```python
from build123d import *

# Parameters (mm, degrees)
BOSS_EXTRUDE1_DEPTH      = 15
BOSS_EXTRUDE1_DEPTH_BACK = 22.5
SKETCH2_W                = 240
SKETCH2_H                = 40
CUT_EXTRUDE1_REACH       = 130.477
SKETCH3_W                = 16
SKETCH3_H                = 2.2
SKETCH3_H_2              = 2.5
SKETCH5_W                = 240
SKETCH5_H                = 40
CUT_EXTRUDE2_DEPTH       = 8
SKETCH6_W                = 20
SKETCH6_H                = 30
BOSS_EXTRUDE2_DEPTH      = 75
CUT_EXTRUDE3_REACH       = 161.707
SKETCH8_W                = 10
SKETCH8_H                = 4.8
SKETCH8_H_2              = 4.5
SKETCH9_R                = 2.1
CUT_EXTRUDE4_DEPTH       = 4.4
SKETCH11_R               = 1.55
CUT_EXTRUDE5_DEPTH       = 11
SKETCH10_R               = 1.55
CUT_EXTRUDE6_DEPTH       = 11
SKETCH12_R               = 2.1
CUT_EXTRUDE7_DEPTH       = 4.4
SKETCH13_R               = 1.65
CUT_EXTRUDE8_DEPTH       = 11
SKETCH14_W               = 18
SKETCH14_H               = 12
CUT_EXTRUDE9_DEPTH       = 29.5
SKETCH15_W               = 10
SKETCH15_H               = 14
CUT_EXTRUDE10_DEPTH      = 20
BOSS_EXTRUDE3_DEPTH      = 10
BOSS_EXTRUDE3_DEPTH_BACK = 50
CUT_EXTRUDE11_REACH      = 163.927
SKETCH18_W               = 89.999903017
SKETCH18_H               = 5
SKETCH18_W_2             = 6.000219265
SKETCH18_W_3             = 65.999877718
SKETCH20_W               = 11
SKETCH20_H               = 12
CUT_EXTRUDE12_DEPTH      = 7
SKETCH21_W               = 8
SKETCH21_H               = 0.5
CUT_EXTRUDE13_DEPTH      = 2
SKETCH22_W               = 8
SKETCH22_H               = 1
CUT_EXTRUDE14_DEPTH      = 2
CUT_EXTRUDE15_REACH      = 163.927
SKETCH23_W               = 11
SKETCH23_H               = 8


with BuildPart() as part:
    # Sketch2 → Boss-Extrude1 (new, two sides: drawn at the far end of the back side and taken through both)
    with BuildSketch(Plane(origin=(0, 0, 0), x_dir=(1, 0, 0), z_dir=(0, 1, 0)).offset(-BOSS_EXTRUDE1_DEPTH_BACK)):
        Rectangle(SKETCH2_W, SKETCH2_H)
    extrude(amount=BOSS_EXTRUDE1_DEPTH + BOSS_EXTRUDE1_DEPTH_BACK)

    # Sketch3 → Cut-Extrude1 (cut, up to next)
    with BuildSketch(Plane.XY.offset(20), mode=Mode.PRIVATE) as cut_extrude1_sk1:
        with Locations((-107, 1.1)):
            Rectangle(SKETCH3_W, SKETCH3_H)
    cut_extrude1_tool1 = extrude(cut_extrude1_sk1.sketch, amount=-CUT_EXTRUDE1_REACH, mode=Mode.PRIVATE) & part.part
    # Sketch3 → Cut-Extrude1 (cut, up to next)
    with BuildSketch(Plane.XY.offset(20), mode=Mode.PRIVATE) as cut_extrude1_sk2:
        with Locations((8.999903017, 1.25)):
            Rectangle(SKETCH3_W, SKETCH3_H_2)
    cut_extrude1_tool2 = extrude(cut_extrude1_sk2.sketch, amount=-CUT_EXTRUDE1_REACH, mode=Mode.PRIVATE) & part.part
    # Sketch3 → Cut-Extrude1 (cut, up to next)
    with BuildSketch(Plane.XY.offset(20), mode=Mode.PRIVATE) as cut_extrude1_sk3:
        with Locations((100.999780735, 1.1)):
            Rectangle(SKETCH3_W, SKETCH3_H)
    cut_extrude1_tool3 = extrude(cut_extrude1_sk3.sketch, amount=-CUT_EXTRUDE1_REACH, mode=Mode.PRIVATE) & part.part
    add(cut_extrude1_tool1.solids().sort_by_distance((-107, 1.1, 20))[0], mode=Mode.SUBTRACT)
    add(cut_extrude1_tool2.solids().sort_by_distance((8.999903, 1.25, 20))[0], mode=Mode.SUBTRACT)
    add(cut_extrude1_tool3.solids().sort_by_distance((100.999781, 1.1, 20))[0], mode=Mode.SUBTRACT)

    # Sketch5 → Cut-Extrude2 (cut)
    with BuildSketch(Plane(origin=(0, 15, 0), x_dir=(1, 0, 0), z_dir=(0, 1, 0))):
        Rectangle(SKETCH5_W, SKETCH5_H)
    extrude(amount=-CUT_EXTRUDE2_DEPTH, mode=Mode.SUBTRACT)

    # Sketch6 → Boss-Extrude2 (add)
    with BuildSketch(Plane.XZ.offset(22.5)):
        with Locations((-70, 0)):
            Rectangle(SKETCH6_W, SKETCH6_H)
    extrude(amount=BOSS_EXTRUDE2_DEPTH)

    # Sketch8 → Cut-Extrude3 (cut, up to next)
    with BuildSketch(Plane.XY.offset(20), mode=Mode.PRIVATE) as cut_extrude3_sk1:
        with Locations((-107, 4.6)):
            Rectangle(SKETCH8_W, SKETCH8_H)
    cut_extrude3_tool1 = extrude(cut_extrude3_sk1.sketch, amount=-CUT_EXTRUDE3_REACH, mode=Mode.PRIVATE) & part.part
    # Sketch8 → Cut-Extrude3 (cut, up to next)
    with BuildSketch(Plane.XY.offset(20), mode=Mode.PRIVATE) as cut_extrude3_sk2:
        with Locations((8.999903017, 4.75)):
            Rectangle(SKETCH8_W, SKETCH8_H_2)
    cut_extrude3_tool2 = extrude(cut_extrude3_sk2.sketch, amount=-CUT_EXTRUDE3_REACH, mode=Mode.PRIVATE) & part.part
    # Sketch8 → Cut-Extrude3 (cut, up to next)
    with BuildSketch(Plane.XY.offset(20), mode=Mode.PRIVATE) as cut_extrude3_sk3:
        with Locations((100.999780735, 4.6)):
            Rectangle(SKETCH8_W, SKETCH8_H)
    cut_extrude3_tool3 = extrude(cut_extrude3_sk3.sketch, amount=-CUT_EXTRUDE3_REACH, mode=Mode.PRIVATE) & part.part
    add(cut_extrude3_tool1.solids().sort_by_distance((-107, 4.6, 20))[0], mode=Mode.SUBTRACT)
    add(cut_extrude3_tool2.solids().sort_by_distance((8.999903, 4.75, 20))[0], mode=Mode.SUBTRACT)
    add(cut_extrude3_tool3.solids().sort_by_distance((100.999781, 4.6, 20))[0], mode=Mode.SUBTRACT)

    # Sketch9 → Cut-Extrude4 (cut)
    with BuildSketch(Plane(origin=(0, 0, 0), x_dir=(1, 0, 0), z_dir=(0, 1, 0))):
        with Locations(Location((-107, 0, 0), (0, 0, 270))):
            Circle(SKETCH9_R)
        with Locations(Location((100.999780735, 0, 0), (0, 0, 270))):
            Circle(SKETCH9_R)
    extrude(amount=-CUT_EXTRUDE4_DEPTH, mode=Mode.SUBTRACT)

    # Sketch11 → Cut-Extrude5 (cut)
    with BuildSketch(Plane(origin=(0, -4.4, 0), x_dir=(1, 0, 0), z_dir=(0, 1, 0))):
        with Locations(Location((100.999780735, 0, 0), (0, 0, 270))):
            Circle(SKETCH11_R)
    extrude(amount=-CUT_EXTRUDE5_DEPTH, mode=Mode.SUBTRACT)

    # Sketch10 → Cut-Extrude6 (cut)
    with BuildSketch(Plane(origin=(0, -4.4, 0), x_dir=(1, 0, 0), z_dir=(0, 1, 0))):
        with Locations(Location((-107, 0, 0), (0, 0, 270))):
            Circle(SKETCH10_R)
    extrude(amount=-CUT_EXTRUDE6_DEPTH, mode=Mode.SUBTRACT)

    # Sketch12 → Cut-Extrude7 (cut)
    with BuildSketch(Plane(origin=(0, 0, 0), x_dir=(1, 0, 0), z_dir=(0, 1, 0))):
        with Locations(Location((10.715225152, -11.813940745, 0), (0, 0, 270))):
            Circle(SKETCH12_R)
        with Locations(Location((10.75, 12, 0), (0, 0, 270))):
            Circle(SKETCH12_R)
    extrude(amount=-CUT_EXTRUDE7_DEPTH, mode=Mode.SUBTRACT)

    # Sketch13 → Cut-Extrude8 (cut)
    with BuildSketch(Plane(origin=(0, -4.4, 0), x_dir=(1, 0, 0), z_dir=(0, 1, 0))):
        with Locations(Location((10.715225152, -11.813940745, 0), (0, 0, 270))):
            Circle(SKETCH13_R)
        with Locations(Location((10.75, 12, 0), (0, 0, 270))):
            Circle(SKETCH13_R)
    extrude(amount=-CUT_EXTRUDE8_DEPTH, mode=Mode.SUBTRACT)

    # Sketch14 → Cut-Extrude9 (cut)
    with BuildSketch(Plane(origin=(0, 7, 0), x_dir=(1, 0, 0), z_dir=(0, 1, 0))):
        with Locations((-16.000096983, 0)):
            Rectangle(SKETCH14_W, SKETCH14_H)
        with Locations((33.999903017, 0)):
            Rectangle(SKETCH14_W, SKETCH14_H)
    extrude(amount=-CUT_EXTRUDE9_DEPTH, mode=Mode.SUBTRACT)

    # Sketch15 → Cut-Extrude10 (cut)
    with BuildSketch(Plane.ZY.offset(80)):
        with Locations((0, -29.5)):
            Rectangle(SKETCH15_W, SKETCH15_H)
    extrude(amount=-CUT_EXTRUDE10_DEPTH, mode=Mode.SUBTRACT)

    # Sketch17 → Boss-Extrude3 (add, two sides: drawn at the far end of the back side and taken through both)
    with BuildSketch(Plane.XY.offset(20).offset(-BOSS_EXTRUDE3_DEPTH_BACK)):
        Polygon((-120, 7), (-120, -22.5), (-94, -22.5), (-94, 7), (-102, 7), (-102, 2.2), (-99, 2.2), (-99, 0), (-115, 0), (-115, 2.2), (-112, 2.2), (-112, 7), align=None)
        Polygon((21.999903017, 7), (21.999903017, -22.5), (-4.000096983, -22.5), (-4.000096983, 7), (3.999903017, 7), (3.999903017, 2.5), (0.999903017, 2.5), (0.999903017, 0), (16.999903017, 0), (16.999903017, 2.5), (13.999903017, 2.5), (13.999903017, 7), align=None)
        Polygon((87.999780735, 7), (87.999780735, -22.5), (113.999780735, -22.5), (113.999780735, 7), (105.999780735, 7), (105.999780735, 2.2), (108.999780735, 2.2), (108.999780735, 0), (92.999780735, 0), (92.999780735, 2.2), (95.999780735, 2.2), (95.999780735, 7), align=None)
    extrude(amount=BOSS_EXTRUDE3_DEPTH + BOSS_EXTRUDE3_DEPTH_BACK)

    # Sketch18 → Cut-Extrude11 (cut, up to next)
    with BuildSketch(Plane(origin=(0, 7, 0), x_dir=(1, 0, 0), z_dir=(0, 1, 0)), mode=Mode.PRIVATE) as cut_extrude11_sk1:
        with Locations((-49.000048492, -17.5)):
            Rectangle(SKETCH18_W, SKETCH18_H)
    cut_extrude11_tool1 = extrude(cut_extrude11_sk1.sketch, amount=-CUT_EXTRUDE11_REACH, mode=Mode.PRIVATE) & part.part
    # Sketch18 → Cut-Extrude11 (cut, up to next)
    with BuildSketch(Plane(origin=(0, 7, 0), x_dir=(1, 0, 0), z_dir=(0, 1, 0)), mode=Mode.PRIVATE) as cut_extrude11_sk2:
        with Locations((116.999890368, -17.5)):
            Rectangle(SKETCH18_W_2, SKETCH18_H)
    cut_extrude11_tool2 = extrude(cut_extrude11_sk2.sketch, amount=-CUT_EXTRUDE11_REACH, mode=Mode.PRIVATE) & part.part
    # Sketch18 → Cut-Extrude11 (cut, up to next)
    with BuildSketch(Plane(origin=(0, 7, 0), x_dir=(1, 0, 0), z_dir=(0, 1, 0)), mode=Mode.PRIVATE) as cut_extrude11_sk3:
        with Locations((-49.000048492, 17.5)):
            Rectangle(SKETCH18_W, SKETCH18_H)
    cut_extrude11_tool3 = extrude(cut_extrude11_sk3.sketch, amount=-CUT_EXTRUDE11_REACH, mode=Mode.PRIVATE) & part.part
    # Sketch18 → Cut-Extrude11 (cut, up to next)
    with BuildSketch(Plane(origin=(0, 7, 0), x_dir=(1, 0, 0), z_dir=(0, 1, 0)), mode=Mode.PRIVATE) as cut_extrude11_sk4:
        with Locations((54.999841876, -17.5)):
            Rectangle(SKETCH18_W_3, SKETCH18_H)
    cut_extrude11_tool4 = extrude(cut_extrude11_sk4.sketch, amount=-CUT_EXTRUDE11_REACH, mode=Mode.PRIVATE) & part.part
    # Sketch18 → Cut-Extrude11 (cut, up to next)
    with BuildSketch(Plane(origin=(0, 7, 0), x_dir=(1, 0, 0), z_dir=(0, 1, 0)), mode=Mode.PRIVATE) as cut_extrude11_sk5:
        with Locations((116.999890368, 17.5)):
            Rectangle(SKETCH18_W_2, SKETCH18_H)
    cut_extrude11_tool5 = extrude(cut_extrude11_sk5.sketch, amount=-CUT_EXTRUDE11_REACH, mode=Mode.PRIVATE) & part.part
    # Sketch18 → Cut-Extrude11 (cut, up to next)
    with BuildSketch(Plane(origin=(0, 7, 0), x_dir=(1, 0, 0), z_dir=(0, 1, 0)), mode=Mode.PRIVATE) as cut_extrude11_sk6:
        with Locations((54.999841876, 17.5)):
            Rectangle(SKETCH18_W_3, SKETCH18_H)
    cut_extrude11_tool6 = extrude(cut_extrude11_sk6.sketch, amount=-CUT_EXTRUDE11_REACH, mode=Mode.PRIVATE) & part.part
    add(cut_extrude11_tool1.solids().sort_by_distance((-49.000048, 7, 17.5))[0], mode=Mode.SUBTRACT)
    add(cut_extrude11_tool2.solids().sort_by_distance((116.99989, 7, 17.5))[0], mode=Mode.SUBTRACT)
    add(cut_extrude11_tool3.solids().sort_by_distance((-49.000048, 7, -17.5))[0], mode=Mode.SUBTRACT)
    add(cut_extrude11_tool4.solids().sort_by_distance((54.999842, 7, 17.5))[0], mode=Mode.SUBTRACT)
    add(cut_extrude11_tool5.solids().sort_by_distance((116.99989, 7, -17.5))[0], mode=Mode.SUBTRACT)
    add(cut_extrude11_tool6.solids().sort_by_distance((54.999842, 7, -17.5))[0], mode=Mode.SUBTRACT)

    # Sketch20 → Cut-Extrude12 (cut)
    with BuildSketch(Plane(origin=(0, 7, 0), x_dir=(1, 0, 0), z_dir=(0, 1, 0))):
        with Locations((-1.500096983, 0)):
            Rectangle(SKETCH20_W, SKETCH20_H)
    extrude(amount=-CUT_EXTRUDE12_DEPTH, mode=Mode.SUBTRACT)

    # Sketch21 → Cut-Extrude13 (cut)
    with BuildSketch(Plane(origin=(0, 7, 0), x_dir=(1, 0, 0), z_dir=(0, 1, 0))):
        with Locations((-98, -0.25)):
            Rectangle(SKETCH21_W, SKETCH21_H)
        with Locations((-98, 0.25)):
            Rectangle(SKETCH21_W, SKETCH21_H)
    extrude(amount=-CUT_EXTRUDE13_DEPTH, mode=Mode.SUBTRACT)

    # Sketch22 → Cut-Extrude14 (cut)
    with BuildSketch(Plane(origin=(0, 7, 0), x_dir=(1, 0, 0), z_dir=(0, 1, 0))):
        with Locations((91.999780735, 0)):
            Rectangle(SKETCH22_W, SKETCH22_H)
    extrude(amount=-CUT_EXTRUDE14_DEPTH, mode=Mode.SUBTRACT)

    # Cut-Extrude15: up to this face of the body (flat: up to its plane)
    cut_extrude15_end = Plane(part.part.faces().sort_by_distance((7.908993926, 0, 0))[0])
    # Sketch23 → Cut-Extrude15 (cut, up to the picked face)
    with BuildSketch(Plane(origin=(0, 7, 0), x_dir=(1, 0, 0), z_dir=(0, 1, 0)), mode=Mode.PRIVATE) as cut_extrude15_sk1:
        with Locations((19.499903017, 0)):
            Rectangle(SKETCH23_W, SKETCH23_H)
    cut_extrude15_tool1 = split(extrude(cut_extrude15_sk1.sketch, amount=-CUT_EXTRUDE15_REACH, mode=Mode.PRIVATE), bisect_by=cut_extrude15_end, keep=Keep.BOTH, mode=Mode.PRIVATE)
    add(cut_extrude15_tool1.solids().sort_by(Axis((19.499903, 7, 0), (0, -1, 0)))[0], mode=Mode.SUBTRACT)


solid = part.part
```
Could you check a few things on this model? Use its own coordinates, in mm. A direction names the side the tool comes from. Coordinates: 2 decimals unless noted, no trailing zeros. Order: outer loops, then holes, each group sorted by start corner. A loop starts at its lowest first (then second) coordinate and runs counter-clockwise, first axis right, second up. Notation, with made-up numbers: M 46.5,25 L 55.5,25 A23 cw 55.5,56 Z; hole C 39,-19.5 d6. An arc over 180 degrees is marked long. Use a Markdown table: item, result. Add a question column.
Q1. I want a section at B-B on y = -3. Give the number of separate pieces and of enclosed holes in the cut face, then the cut area to 3 significant figures.
Q2. I want a section at A-A on x = 30. List the corners of the cut face in (y, z) for me.
Q3. If I drill on L1, parallel to X at y = -12, z = -2; L2, parallel to X at y = -9, z = 19.5; L3, parallel to Y at x = 106.5, z = 1.5, over which ranges is the centre line in solid material (lowest first)?
Q4. I want a section at D-D on y = -54.5. List the corners of the cut face in (x, z) for me.
Q5. Which directions (+Z, -Z, +X, -X, +Y, -Y) give clear straight access to the entire face, cutting with the end or side of a thin tool? Please do faces 1 (the flat face through (-25, -8, 0)), 2 (the flat face through (-94, -8, -23)), 3 (the flat face through (-80, -59, 0)).
Q6. We'd pull the mould along Z, two halves only. Please class faces 4 (the flat face through (101, -8, -30)), 5 (the flat face through (-120, -8, 0)), 6 (the flat face through (-70, -30, -5)): pulls with the +Z half, pulls with the -Z half, needs draft (parallel to the pull), parting line crosses it, or undercut.
Q7. I'm going to push flat-ended pins straight in: pin 1 (0.5 mm diameter, centred on x = -100, z = 0, fed in from +Y); pin 2 (0.9 mm diameter, centred on x = -100.5, z = 4.5, fed in from -Y); pin 3 (3 mm diameter, centred on x = 35.5, y = -10, fed in from -Z). Where does each tip first touch, or does it pass through?
Checked values:
| question | item | result |
|---|---|---|
| 1 | separate pieces | 1 |
| 1 | enclosed holes | 2 |
| 1 | area | 9,110 mm² |
| 2 | outline | M -22.5,-15 L 7,-15 L 7,-6 L -22.5,-6 Z; M -22.5,6 L 7,6 L 7,15 L -22.5,15 Z |
| 3 | L1 | -120 to -25, -7 to 25, 43 to 120 |
| 3 | L2 | -120 to -94, -4 to 22, 88 to 114 |
| 3 | L3 | -22.5 to 0, 2.2 to 7 |
| 4 | outline | M -80,-15 L -60,-15 L -60,15 L -80,15 Z |
| 5 | face 1 | +Y, -Y |
| 5 | face 2 | -Z, +Y, -Y |
| 5 | face 3 | +Z, -Z, -X, -Y |
| 6 | face 4 | pulls with the -Z half |
| 6 | face 5 | needs draft |
| 6 | face 6 | undercut |
| 7 | pin 1 | y = 5 |
| 7 | pin 2 | y = -22.5 |
| 7 | pin 3 | z = -15 |
